from build123d import *

# Parameters (mm, degrees)
F0_W     = 1000
F0_H     = 500
F1_DEPTH = 25.4
F2_T     = -2.54
F3_W     = 30
F3_H     = 30
F4_DEPTH = 1000
F6_W     = 994.92
F6_H     = 434.92
F7_DEPTH = 25.4


with BuildPart() as f1:
    # F0 (on Top) → F1 (new body)
    with BuildSketch(Plane.XY):
        Rectangle(F0_W, F0_H)
    extrude(amount=F1_DEPTH)

    # F2
    f2_openings = [f1.faces().sort_by_distance(p)[0] for p in [
        (0, 0, 0),
    ]]
    offset(amount=F2_T, openings=f2_openings)

    # F3 (on face) → F4 (join)
    with BuildSketch(Plane(origin=(0, 0, 22.86), x_dir=(1, 0, 0), z_dir=(0, 0, -1))):
        with Locations((-482.46, 232.46)):
            Rectangle(F3_W, F3_H)
        with Locations((-482.46, -232.46)):
            Rectangle(F3_W, F3_H)
        with Locations((482.46, 232.46)):
            Rectangle(F3_W, F3_H)
        with Locations((482.46, -232.46)):
            Rectangle(F3_W, F3_H)
    extrude(amount=F4_DEPTH)

    # F6 (on offset) → F7 (join)
    with BuildSketch(Plane(origin=(0, 0, -877.14), x_dir=(1, 0, 0), z_dir=(0, 0, -1))):
        Rectangle(F6_W, F6_H)
    extrude(amount=-F7_DEPTH)


solid = f1.part
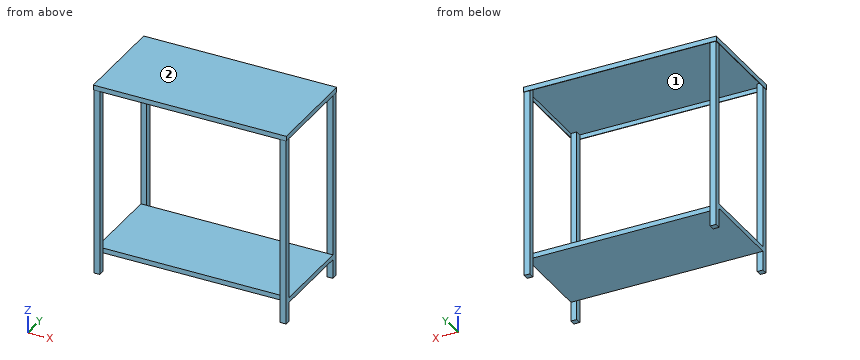
Can you work these out from the model? Positions are in its coordinate system, mm. Face numbers are marked on the shaded views. Coordinates: 2 decimals unless noted, no trailing zeros. Order: outer loops, then holes, each group sorted by start corner. A loop starts at its lowest first (then second) coordinate and runs counter-clockwise, first axis right, second up. Notation, with made-up numbers: (12.25, 59) - (58.25, 59) arc R21 ccw to (58.25, 70) - close; hole circle Ø7 at (42, 47.5). An arc over 180 degrees is marked (long way). Answer as a JSON object with one key per item and string values. Group by question number.
Q1. Imagine slicing it at A-A (z = -318.5). Please give me the cut outline in (x, y).
Q2. Will these pins go through, and if not, where does the flat tip stop? P1, Ø3, axis at y = 96.5, z = -853, coming from the -X side; P2, Ø7.5, axis at x = -189.5, z = -869, coming from the -Y side; P3, Ø12.5, axis at x = -76, z = -864, coming from the +Y side.
Q3. Imagine slicing it at B-B (x = 319.5). Please give me the cut outline in (y, z), and give its area (3 significant figures).
Q4. I need wall thicknesses on line 1 (Z direction, x = 45, y = -26); line 2 (X direction, y = 217.5, z = -806.5); line 3 (Z direction, x = 227, y = -217.5). Which ranges of each line are inside material? Lowest first, please. Write a range as from..to.
Q5. Imagine slicing it at C-C (y = 19.5). Please give me the cut outline in (x, z), and give its area (3 significant figures).
Q6. We'd pull the mould along X, two halves only. Please class the marked faces 1 and 2: +X half, -X half, draft (parallel to the pull), parting line (faces both ways), or undercut.
Determined:
{
 "1": {"outline": "(-497.46, -247.46) - (-467.46, -247.46) - (-467.46, -217.46) - (-497.46, -217.46) - close; (-497.46, 217.46) - (-467.46, 217.46) - (-467.46, 247.46) - (-497.46, 247.46) - close; (467.46, -247.46) - (497.46, -247.46) - (497.46, -217.46) - (467.46, -217.46) - close; (467.46, 217.46) - (497.46, 217.46) - (497.46, 247.46) - (467.46, 247.46) - close"},
 "2": {"P1": "stops at x = -497.46", "P2": "stops at y = -217.46", "P3": "stops at y = 217.46"},
 "3": {"outline": "(-250, 0) - (-247.46, 0) - (-247.46, 22.86) - (247.46, 22.86) - (247.46, 0) - (250, 0) - (250, 25.4) - (-250, 25.4) - close; (-217.46, -877.14) - (217.46, -877.14) - (217.46, -851.74) - (-217.46, -851.74) - close", "area": "12,400 mm2"},
 "4": {"line 1": "z = -877.14..-851.74, 22.86..25.4", "line 2": "x = -497.46..-467.46, 467.46..497.46", "line 3": "z = 22.86..25.4"},
 "5": {"outline": "(-500, 0) - (-497.46, 0) - (-497.46, 22.86) - (497.46, 22.86) - (497.46, 0) - (500, 0) - (500, 25.4) - (-500, 25.4) - close; (-497.46, -877.14) - (497.46, -877.14) - (497.46, -851.74) - (-497.46, -851.74) - close", "area": "27,900 mm2"},
 "6": {"face 1": "undercut", "face 2": "draft"}
}
